```python
from build123d import *

# Parameters (mm, degrees)
SKETCH_1_W               = 300
SKETCH_1_H               = 300
EXTRUDE_1_DEPTH          = 3
SKETCH_2_R               = 1.5
CUT_EXTRUDE_1_DEPTH      = 213.153246499
FILLET_1_R               = 10
SKETCH_3_R               = 5
CUT_EXTRUDE_2_DEPTH      = 213.153246499
MIRROR_3_COPY_1_SKETCH_R = 5
MIRROR_3_COPY_1_DEPTH    = 213.153246499
SKETCH_4_R               = 5
CUT_EXTRUDE_3_DEPTH      = 213.153246499
SKETCH_5_R               = 3
CUT_EXTRUDE_4_DEPTH      = 213.153246499
SKETCH_6_R               = 3
CUT_EXTRUDE_5_DEPTH      = 213.153246499


with BuildPart() as part:
    # 草图1 → 凸台-拉伸1 (new body)
    with BuildSketch(Plane.XY):
        Rectangle(SKETCH_1_W, SKETCH_1_H)
    extrude(amount=EXTRUDE_1_DEPTH)

    # 草图2 → 切除-拉伸1 (cut, through all)
    with BuildSketch(Plane.XY.offset(3)):
        with Locations((103, 90)):
            Circle(SKETCH_2_R)
        with Locations((127, 90)):
            Circle(SKETCH_2_R)
        with Locations((103, 60)):
            Circle(SKETCH_2_R)
        with Locations((127, 60)):
            Circle(SKETCH_2_R)
    cut_extrude_1 = extrude(amount=-CUT_EXTRUDE_1_DEPTH, mode=Mode.SUBTRACT)

    # 镜向1: 切除-拉伸1 across plane
    add(cut_extrude_1.mirror(Plane(origin=(0, 0, 0), x_dir=(0, 0, 1), z_dir=(1, 0, 0))), mode=Mode.SUBTRACT)

    # 圆角1
    fillet_1_edges = [part.edges().sort_by_distance(p)[0] for p in [
        (-150, 150, 1.5),
        (150, 150, 1.5),
        (150, -150, 1.5),
        (-150, -150, 1.5),
    ]]
    fillet(fillet_1_edges, radius=FILLET_1_R)

    # 草图3 → 切除-拉伸2 (cut, through all)
    with BuildSketch(Plane.XY.offset(3)):
        with Locations((-130, 130)):
            Circle(SKETCH_3_R)
    cut_extrude_2 = extrude(amount=-CUT_EXTRUDE_2_DEPTH, mode=Mode.SUBTRACT)

    # 镜向2: 切除-拉伸2 across plane
    add(cut_extrude_2.mirror(Plane(origin=(0, 0, 0), x_dir=(0, 0, 1), z_dir=(1, 0, 0))), mode=Mode.SUBTRACT)

    # 镜向3: 切除-拉伸2 across plane
    add(cut_extrude_2.mirror(Plane.ZX), mode=Mode.SUBTRACT)

    # 镜向3 copy 1 sketch → 镜向3 copy 1 (cut, through all)
    with BuildSketch(Plane(origin=(0, 0, 3), x_dir=(-1, 0, 0), z_dir=(0, 0, 1))):
        with Locations((-130, 130)):
            Circle(MIRROR_3_COPY_1_SKETCH_R)
    extrude(amount=-MIRROR_3_COPY_1_DEPTH, mode=Mode.SUBTRACT)

    # 草图4 → 切除-拉伸3 (cut, through all)
    with BuildSketch(Plane.XY.offset(3)):
        with Locations((-70, 75)):
            Circle(SKETCH_4_R)
        with Locations((70, 75)):
            Circle(SKETCH_4_R)
    extrude(amount=-CUT_EXTRUDE_3_DEPTH, mode=Mode.SUBTRACT)

    # 草图5 → 切除-拉伸4 (cut, through all)
    with BuildSketch(Plane.XY.offset(3)):
        with Locations((-130, -100)):
            Circle(SKETCH_5_R)
        with Locations((-130, -60)):
            Circle(SKETCH_5_R)
        with Locations((-100, -60)):
            Circle(SKETCH_5_R)
        with Locations((-100, -100)):
            Circle(SKETCH_5_R)
    cut_extrude_4 = extrude(amount=-CUT_EXTRUDE_4_DEPTH, mode=Mode.SUBTRACT)

    # 镜向4: 切除-拉伸4 across plane
    add(cut_extrude_4.mirror(Plane(origin=(0, 0, 0), x_dir=(0, 0, 1), z_dir=(1, 0, 0))), mode=Mode.SUBTRACT)

    # 草图6 → 切除-拉伸5 (cut, through all)
    with BuildSketch(Plane.XY.offset(3)):
        with Locations((-15, -60)):
            Circle(SKETCH_6_R)
        with Locations((15, -60)):
            Circle(SKETCH_6_R)
        with Locations((-15, -100)):
            Circle(SKETCH_6_R)
        with Locations((15, -100)):
            Circle(SKETCH_6_R)
    extrude(amount=-CUT_EXTRUDE_5_DEPTH, mode=Mode.SUBTRACT)


solid = part.part
```
Input: part model. Units: mm. Frame: model coordinates. Round coordinates to 2 decimals unless told otherwise and drop trailing zeros. Order: outer loops, then holes, each group sorted by start corner. A loop starts at its lowest first (then second) coordinate and runs counter-clockwise, first axis right, second up. Notation, with made-up numbers: (-15, -14.5) - (24, -14.5) arc R8 ccw to (24, -6.5) - close; hole circle Ø5 at (61.25, 68.25). An arc over 180 degrees is marked (long way). Answer in a Markdown table with one row per item.
Item 1: Section query A-A (y = 75). Return the cut outline in (x, z), then the cut area to 3 significant figures.
Model answer:
| item | result |
|---|---|
| outline | (-150, 0) - (-75, 0) - (-75, 3) - (-150, 3) - close; (-65, 0) - (65, 0) - (65, 3) - (-65, 3) - close; (75, 0) - (150, 0) - (150, 3) - (75, 3) - close |
| area | 840 mm² |
Item 2: Section query B-B (x = -70). Return the cut outline in (y, z).
Model answer:
| item | result |
|---|---|
| outline | (-150, 0) - (70, 0) - (70, 3) - (-150, 3) - close; (80, 0) - (150, 0) - (150, 3) - (80, 3) - close |
Item 3: Mould query, pull axis X, two halves, no side actions, for faces 1 (the cylindrical face through (-147.15, 146.99, 1.52)), 2 (the cylindrical face through (146.99, -147.15, 1.52)), 3 (the cylindrical face through (-125.381, -128.085, 1.521)). Classes: released by +X, released by -X, zero draft, split by the parting line, or undercut.
Model answer:
| item | result |
|---|---|
| face 1 | released by -X |
| face 2 | released by +X |
| face 3 | undercut |
Item 4: Line query: line 1 (X direction, y = 90, z = 2.1); line 2 (X direction, y = -130, z = 1.7); line 3 (Y direction, x = -15, z = 1.8). Output: solid intervals per line, ascending.
Model answer:
| item | result |
|---|---|
| line 1 | x = -150 to -128.5, -125.5 to -104.5, -101.5 to 101.5, 104.5 to 125.5, 128.5 to 150 |
| line 2 | x = -150 to -135, -125 to 125, 135 to 150 |
| line 3 | y = -150 to -103, -97 to -63, -57 to 150 |
